Input: dimensioned drawing with shaded views. Units: mm. Origin: part minimum x, y, z. Give positions to 0.01 mm unless a question says otherwise; leave off trailing zeros. Write each loop counter-clockwise with the first axis right and the second up, starting at its lowest first coordinate (ties: lowest second). Pieces come first, ordered by that corner, then holes. Notation, with made-up numbers: (-22, 84) -> (0, 84) arc R14 ccw to (0, 88) -> close; hole circle Ø10 at (-21, 86.5). An arc over 180 degrees is marked (long way). Return JSON: item names as keys, results as strings. Group by question number.
Item 1: Pin query (flat end, axial travel): P1, Ø0.9, axis at x = 8, z = 1.5, coming from the +Y side; P2, Ø0.9, axis at x = 8.5, z = 1, coming from the -Y side. Return the tip coordinate at first contact, or that it passes through.
Item 2: Section A-A, the plane x = 25. Return loops of the section in (y, z).
Item 3: Section C-C, the plane z = 1.7. Return loops of the section in (x, y), then the cut area to 3 significant figures.
Item 4: Section B-B, the plane y = 12.5. Return loops of the section in (x, z), then the cut area to 3 significant figures.
Item 5: Line query: line 1 (X direction, y = 1.5, z = 1.05); line 2 (Y direction, x = 25, z = 1.85); line 3 (Y direction, x = 44.5, z = 2). Output: solid intervals per line, ascending. Write a range as [from, to].
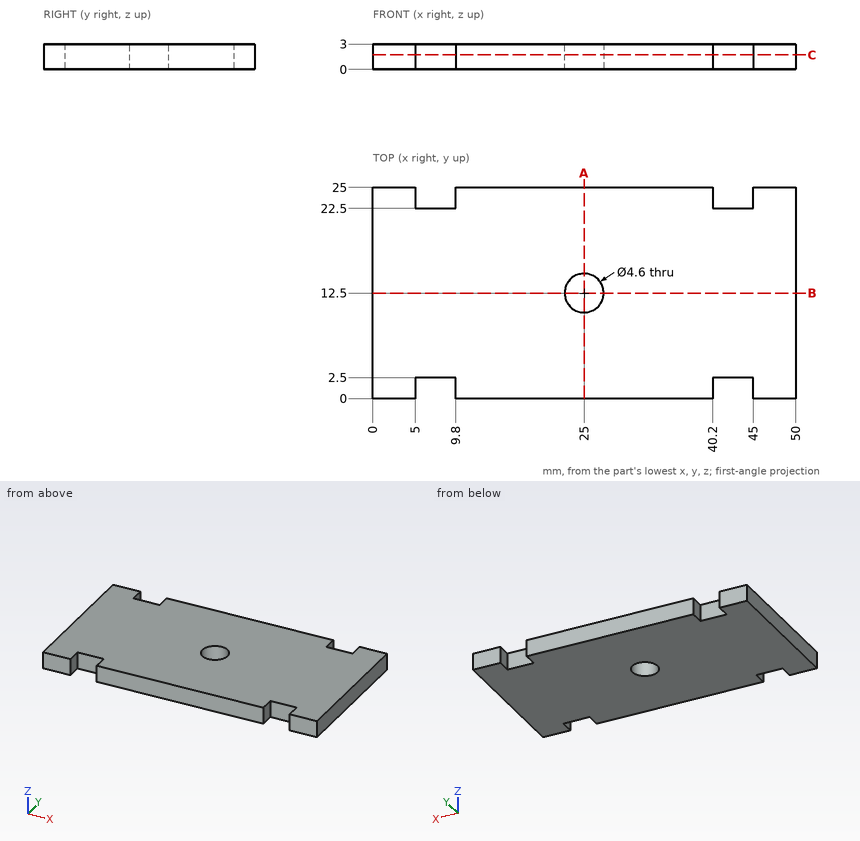
Answer below:
{
 "1": {"P1": "stops at y = 22.5", "P2": "stops at y = 2.5"},
 "2": {"outline": "(0, 0) -> (10.2, 0) -> (10.2, 3) -> (0, 3) -> close; (14.8, 0) -> (25, 0) -> (25, 3) -> (14.8, 3) -> close"},
 "3": {"outline": "(0, 0) -> (5, 0) -> (5, 2.5) -> (9.8, 2.5) -> (9.8, 0) -> (40.2, 0) -> (40.2, 2.5) -> (45, 2.5) -> (45, 0) -> (50, 0) -> (50, 25) -> (45, 25) -> (45, 22.5) -> (40.2, 22.5) -> (40.2, 25) -> (9.8, 25) -> (9.8, 22.5) -> (5, 22.5) -> (5, 25) -> (0, 25) -> close; hole circle Ø4.6 at (25, 12.5)", "area": "1,190 mm2"},
 "4": {"outline": "(0, 0) -> (22.7, 0) -> (22.7, 3) -> (0, 3) -> close; (27.3, 0) -> (50, 0) -> (50, 3) -> (27.3, 3) -> close", "area": "136 mm2"},
 "5": {"line 1": "x = [0, 5], [9.8, 40.2], [45, 50]", "line 2": "y = [0, 10.2], [14.8, 25]", "line 3": "y = [2.5, 22.5]"}
}
